from build123d import *

# Parameters (mm, degrees)
SKETCH_1_R               = 18
EXTRUDE_1_DEPTH          = 8.5
SKETCH_2_R               = 17.95
EXTRUDE_2_DEPTH          = 19
SKETCH_3_R               = 18
EXTRUDE_3_DEPTH          = 5
SKETCH_4_R               = 11
EXTRUDE_4_DEPTH          = 2
SKETCH_5_R               = 5
EXTRUDE_5_DEPTH          = 1
SKETCH_6_R               = 4
EXTRUDE_6_DEPTH          = 17
CUT_EXTRUDE_1_DEPTH      = 1
CUT_EXTRUDE_1_DEPTH_BACK = 15
SKETCH_8_R               = 11
CUT_EXTRUDE_2_DEPTH      = 4
SKETCH_9_R               = 4
CUT_EXTRUDE_3_DEPTH      = 17
SKETCH_10_R              = 1.5
CUT_EXTRUDE_4_DEPTH      = 10
PATTERN_CIRCULAR_1_COUNT = 8
SKETCH_11_R              = 2.5
CUT_EXTRUDE_5_DEPTH      = 3.5
PATTERN_CIRCULAR_2_COUNT = 4


with BuildPart() as part:
    # 草圖1 → 填料-伸長1 (new body)
    with BuildSketch(Plane.XY):
        Circle(SKETCH_1_R)
    extrude(amount=EXTRUDE_1_DEPTH)

    # 草圖2 → 填料-伸長2 (add)
    with BuildSketch(Plane(origin=(0, 0, 0), x_dir=(-1, 0, 0), z_dir=(0, 0, -1))):
        Circle(SKETCH_2_R)
    extrude(amount=EXTRUDE_2_DEPTH)

    # 草圖3 → 填料-伸長3 (add)
    with BuildSketch(Plane(origin=(0, 0, -19), x_dir=(-1, 0, 0), z_dir=(0, 0, -1))):
        Circle(SKETCH_3_R)
    extrude(amount=EXTRUDE_3_DEPTH)

    # 草圖4 → 填料-伸長4 (add)
    with BuildSketch(Plane.XY.offset(8.5)):
        Circle(SKETCH_4_R)
    extrude(amount=EXTRUDE_4_DEPTH)

    # 草圖5 → 填料-伸長5 (add)
    with BuildSketch(Plane.XY.offset(10.5)):
        Circle(SKETCH_5_R)
    extrude(amount=EXTRUDE_5_DEPTH)

    # 草圖6 → 填料-伸長6 (add)
    with BuildSketch(Plane.XY.offset(11.5)):
        Circle(SKETCH_6_R)
    extrude(amount=EXTRUDE_6_DEPTH)

    # 草圖7 → 除料-伸長1 (cut, two sides)
    with BuildSketch(Plane.XY.offset(28.5)) as cut_extrude_1_sk:
        Polygon((-71.543868334, 3), (-2.645751311, 3), (2.645751311, 3), (71.543868334, 3), (71.543868334, 140.796234045), (-71.543868334, 140.796234045), align=None)
    extrude(amount=CUT_EXTRUDE_1_DEPTH, mode=Mode.SUBTRACT)
    extrude(cut_extrude_1_sk.sketch, amount=-CUT_EXTRUDE_1_DEPTH_BACK, mode=Mode.SUBTRACT)

    # 草圖8 → 除料-伸長2 (cut)
    with BuildSketch(Plane(origin=(0, 0, -24), x_dir=(-1, 0, 0), z_dir=(0, 0, -1))):
        Circle(SKETCH_8_R)
    extrude(amount=-CUT_EXTRUDE_2_DEPTH, mode=Mode.SUBTRACT)

    # 草圖9 → 除料-伸長3 (cut)
    with BuildSketch(Plane(origin=(0, 0, -24), x_dir=(-1, 0, 0), z_dir=(0, 0, -1))):
        Circle(SKETCH_9_R)
    extrude(amount=-CUT_EXTRUDE_3_DEPTH, mode=Mode.SUBTRACT)

    # 草圖10 → 除料-伸長4 (cut)
    with BuildSketch(Plane.XY.offset(8.5)):
        with Locations((0, 15)):
            Circle(SKETCH_10_R)
    cut_extrude_4 = extrude(amount=-CUT_EXTRUDE_4_DEPTH, mode=Mode.SUBTRACT)

    # 環狀複製排列1: 除料-伸長4 ×8 about axis
    pattern_circular_1_axis = Axis((0, 0, 0), (0, 0, 1))
    for i in range(1, PATTERN_CIRCULAR_1_COUNT):
        add(cut_extrude_4.rotate(pattern_circular_1_axis, i * 360 / PATTERN_CIRCULAR_1_COUNT), mode=Mode.SUBTRACT)

    # 草圖11 → 除料-伸長5 (cut)
    with BuildSketch(Plane.XY.offset(8.5)):
        with Locations((0, 15)):
            Circle(SKETCH_11_R)
    cut_extrude_5 = extrude(amount=-CUT_EXTRUDE_5_DEPTH, mode=Mode.SUBTRACT)

    # 環狀複製排列2: 除料-伸長5 ×4 about axis
    pattern_circular_2_axis = Axis((0, 0, 0), (0, 0, 1))
    for i in range(1, PATTERN_CIRCULAR_2_COUNT):
        add(cut_extrude_5.rotate(pattern_circular_2_axis, i * 360 / PATTERN_CIRCULAR_2_COUNT), mode=Mode.SUBTRACT)


solid = part.part
Here's how the part is built. I have some questions about the finished solid (model axes, mm). A direction names the side the tool comes from. Coordinates: 2 decimals unless noted, no trailing zeros. Loops run counter-clockwise (first coordinate to the right, second up) from the corner with the lowest first, then second, coordinate; pieces in that order, holes last. Notation, with made-up numbers: (86.5, 83) -> (123.5, 83) arc R7 cw to (123.5, 94) -> close; hole circle Ø6 at (58, -36). An arc over 180 degrees is marked (long way). Use one line per item in the form item = value. Start each with the question number.
(1) On a 3-axis mill with a long thin cutter (end or side, diameter ignored), from which of +Z, -Z, +X, -X, +Y, -Y can I reach the whole of each face in a straight line? I mean faces 5 (the face through (-11, 11, -1.5)), 6 (the face through (-2.343, 17.847, 4.19)), 7 (the face through (0, 0, -7)), 8 (the face through (-17.12, 5.39, -9.37)). Say none if no direction works.
(2) Please list where these lines run through material, in increasing order: line 1 along Y through (x, z) = (0, 3.25); line 2 along Y through (x, z) = (0, 6.7); line 3 along Z through (x, y) = (-13.5, -4).
(3) If we section it at B-B (y = 7.5): Please give me the cut outline in (x, z).
(4) If we section it at C-C (x = -15): Please give me the cut outline in (y, z), then the cut area to 3 significant figures.
(5) If we section it at D-D (z = 17): Please give me the cut outline in (x, y).
(6) If we section it at A-A (z = -15.5): Please give me the cut outline in (x, y).
(7) We'd pull the mould along Y, two halves only. Please class faces 1 (the face through (2, -5, 10.5)), 2 (the face through (0, 3, 21)), 3 (the face through (0, -5, -20)), 4 (the face through (-0.867, -3.905, 19.881)): pulls with the +Y half, pulls with the -Y half, needs draft (parallel to the pull), parting line crosses it, or undercut.
(8) Will these pins go through, and if not, where does the flat tip stop? pin 1 (5.5 mm diameter, centred on x = 0.5, y = 15.5, fed in from +Z); pin 2 (1.5 mm diameter, centred on x = -15.5, y = 0.5, fed in from +Z); pin 3 (3 mm diameter, centred on y = 1, z = 10.5, fed in from -X); pin 4 (17.5 mm diameter, centred on x = 2.5, y = 1, fed in from -Z).
Verdict:
q1.face_5 = +Z
q1.face_6 = +Z, -Z
q1.face_7 = -Z
q1.face_8 = none
q2.line_1 = -18 to -16.5, -13.5 to 13.5, 16.5 to 18
q2.line_2 = -18 to -17.5, -12.5 to 12.5, 17.5 to 18
q2.line_3 = -24 to 8.5
q3.outline = (-16.36, -24) -> (-8.05, -24) -> (-8.05, -20) -> (8.05, -20) -> (8.05, -24) -> (16.36, -24) -> (16.36, -19) -> (16.31, -19) -> (16.31, 0) -> (16.36, 0) -> (16.36, 8.5) -> (8.05, 8.5) -> (8.05, 10.5) -> (-8.05, 10.5) -> (-8.05, 8.5) -> (-16.36, 8.5) -> (-16.36, 0) -> (-16.31, 0) -> (-16.31, -19) -> (-16.36, -19) -> close
q4.outline = (-9.95, -24) -> (9.95, -24) -> (9.95, -19) -> (9.86, -19) -> (9.86, 0) -> (9.95, 0) -> (9.95, 8.5) -> (2.5, 8.5) -> (2.5, 5) -> (1.5, 5) -> (1.5, -1.5) -> (-1.5, -1.5) -> (-1.5, 5) -> (-2.5, 5) -> (-2.5, 8.5) -> (-9.95, 8.5) -> (-9.95, 0) -> (-9.86, 0) -> (-9.86, -19) -> (-9.95, -19) -> close
q4.area = 606 mm²
q5.outline = (-2.65, 3) arc R4 ccw (long way) to (2.65, 3) -> close
q6.outline = circle Ø35.9 at (0, 0); hole circle Ø8 at (0, 0)
q7.face_1 = needs draft
q7.face_2 = pulls with the +Y half
q7.face_3 = undercut
q7.face_4 = parting line crosses it
q8.pin_1 = 8.5
q8.pin_2 = -1.5
q8.pin_3 = -11
q8.pin_4 = -24
